For this review, take the finished solid that the model builds, in its own axes (mm). A direction names the side the tool comes from. Coordinates: 2 decimals unless noted, no trailing zeros. Order: outer loops, then holes, each group sorted by start corner. A loop starts at its lowest first (then second) coordinate and runs counter-clockwise, first axis right, second up. Notation, with made-up numbers: (63.5, 3) -> (122.5, 3) arc R13 ccw to (122.5, 28) -> close; hole circle Ø10 at (-35.5, 67). An arc over 180 degrees is marked (long way). Answer as a JSON object with one key per item and string values. Group by question number.
1) Machinability: for faces 4 (the flat face through (6, 7, 3)), 5 (the flat face through (-0.1, 26.5, 0.5)), 6 (the flat face through (0, 12, -6)), which of the approach directions +Z, -Z, +X, -X, +Y, -Y give a long, thin tool a straight path to every point of the face, cutting with its end or side? Answer none if there is none.
2) Add section A-A, the plane z = 2.75. Write out the cut boundary in (x, y).
3) For pin 1 (2 mm diameter, centred on x = 6, y = -6.5, fed in from +Z); pin 2 (2 mm diameter, centred on x = 5.5, y = -6, fed in from -Z); pin 3 (1.6 mm diameter, centred on x = 5.5, y = 5.5, fed in from +Z), all flat-tipped, find the tip position at first contact; note any pin that passes through.
4) Wall thickness on L1, parallel to Y at x = -7, z = -4.25; L2, parallel to X at y = 24, z = 2; L3, parallel to Y at x = -8.25, z = 2: over which ranges is each line inside the solid? List them lowest first.
5) Add section B-B, the plane y = 21. Write out the cut boundary in (x, z), then the cut area to 3 significant figures.
6) Add section D-D, the plane y = -5.5. Write out the cut boundary in (x, z).
7) Draft analysis for pull direction X (two halves, no side actions). For faces 1 (the flat face through (0, 19, -7.5)), 2 (the flat face through (6, -6, -2)), 3 (the flat face through (-12, 0, 0)), state which applies: +X half, -X half, draft (parallel to the pull), parting line (faces both ways), or undercut.
from build123d import *

# Parameters (mm, degrees)
AUFSATZ_LINEAR_AUSTRAGEN1_DEPTH      = 5
AUFSATZ_LINEAR_AUSTRAGEN1_DEPTH_BACK = 5
SKIZZE1_W                            = 24
SKIZZE1_H                            = 24
SKIZZE3_W                            = 15
SKIZZE3_H                            = 15
AUFSATZ_LINEAR_AUSTRAGEN2_DEPTH      = 15
SCHNITT_LINEAR_AUSTRAGEN1_DEPTH      = 10
FASE1_SIZE                           = 1
SCHNITT_LINEAR_START                 = -11
SKIZZE6_W                            = 2
SKIZZE6_H                            = 2
SCHNITT_LINEAR_AUSTRAGEN2_DEPTH      = 12
FASE2_SIZE                           = 1
SKIZZE12_W                           = 15
SKIZZE12_H                           = 15
SCHNITT_LINEAR_AUSTRAGEN4_DEPTH      = 2.5


with BuildPart() as part:
    # Skizze1 → Aufsatz-Linear austragen1 (new, two sides: drawn at the far end of the back side and taken through both)
    with BuildSketch(Plane.XY.offset(-AUFSATZ_LINEAR_AUSTRAGEN1_DEPTH_BACK)):
        Rectangle(SKIZZE1_W, SKIZZE1_H)
    extrude(amount=AUFSATZ_LINEAR_AUSTRAGEN1_DEPTH + AUFSATZ_LINEAR_AUSTRAGEN1_DEPTH_BACK)

    # Skizze3 → Aufsatz-Linear austragen2 (add)
    with BuildSketch(Plane(origin=(0, 12, 0), x_dir=(1, 0, 0), z_dir=(0, 1, 0))):
        Rectangle(SKIZZE3_W, SKIZZE3_H)
    extrude(amount=AUFSATZ_LINEAR_AUSTRAGEN2_DEPTH)

    # Skizze5 → Schnitt-Linear austragen1 (cut)
    with BuildSketch(Plane(origin=(0, 27, 0), x_dir=(1, 0, 0), z_dir=(0, 1, 0))):
        with BuildLine():
            Line((-5.1, 0), (5.1, 0))
            ThreePointArc((5.1, 0), (0, 5.1), (-5.1, 0))
        make_face()
    extrude(amount=-SCHNITT_LINEAR_AUSTRAGEN1_DEPTH, mode=Mode.SUBTRACT)

    # Fase1
    fase1_edges = [part.edges().sort_by_distance(p)[0] for p in [
        (0, 27, -5.1),
        (0, 27, 0),
    ]]
    chamfer(fase1_edges, length=FASE1_SIZE)

    # Skizze6 → Schnitt-Linear austragen2 (cut)
    with BuildSketch(Plane.XY.offset(-3).offset(SCHNITT_LINEAR_START)):
        with Locations((6, 6)):
            Rectangle(SKIZZE6_W, SKIZZE6_H)
        with Locations((6, -6)):
            Rectangle(SKIZZE6_W, SKIZZE6_H)
        with Locations((-6, -6)):
            Rectangle(SKIZZE6_W, SKIZZE6_H)
        with Locations((-6, 6)):
            Rectangle(SKIZZE6_W, SKIZZE6_H)
    schnitt_linear_austragen2 = extrude(amount=SCHNITT_LINEAR_AUSTRAGEN2_DEPTH, mode=Mode.SUBTRACT)

    # Spiegeln1: Schnitt-Linear austragen2 across plane
    add(schnitt_linear_austragen2.mirror(Plane.XY), mode=Mode.SUBTRACT)

    # Fase2
    fase2_edges = [part.edges().sort_by_distance(p)[0] for p in [
        (6, 5, 5),
        (7, 6, 5),
        (6, 7, 5),
        (5, 6, 5),
        (6, -7, 5),
        (7, -6, 5),
        (6, -5, 5),
        (5, -6, 5),
        (-6, -7, 5),
        (-5, -6, 5),
        (-6, -5, 5),
        (-7, -6, 5),
        (-6, 5, 5),
        (-5, 6, 5),
        (-6, 7, 5),
        (-7, 6, 5),
        (6, 7, -5),
        (7, 6, -5),
        (6, 5, -5),
        (5, 6, -5),
        (6, -5, -5),
        (7, -6, -5),
        (6, -7, -5),
        (5, -6, -5),
        (-6, -5, -5),
        (-5, -6, -5),
        (-6, -7, -5),
        (-7, -6, -5),
        (-6, 7, -5),
        (-5, 6, -5),
        (-6, 5, -5),
        (-7, 6, -5),
    ]]
    chamfer(fase2_edges, length=FASE2_SIZE)

    # Skizze12 → Schnitt-Linear austragen4 (cut)
    with BuildSketch(Plane.XY.offset(7.5)):
        with Locations((0, 19.5)):
            Rectangle(SKIZZE12_W, SKIZZE12_H)
    extrude(amount=-SCHNITT_LINEAR_AUSTRAGEN4_DEPTH, mode=Mode.SUBTRACT)


solid = part.part
Output values:
{
 "1": {"face 4": "+Z", "face 5": "+Y", "face 6": "-Z, +X, -X, -Y"},
 "2": {"outline": "(-12, -12) -> (12, -12) -> (12, 12) -> (7.5, 12) -> (7.5, 27) -> (-7.5, 27) -> (-7.5, 12) -> (-12, 12) -> close; hole (-7, -7) -> (-5, -7) -> (-5, -5) -> (-7, -5) -> close; hole (-7, 5) -> (-5, 5) -> (-5, 7) -> (-7, 7) -> close; hole (5, -7) -> (7, -7) -> (7, -5) -> (5, -5) -> close; hole (5, 5) -> (7, 5) -> (7, 7) -> (5, 7) -> close"},
 "3": {"pin 1": "stops at z = 4.5", "pin 2": "stops at z = -4.5", "pin 3": "stops at z = 4.3"},
 "4": {"L1": "y = -12 to -7.25, -4.75 to 4.75, 7.25 to 27", "L2": "x = -7.5 to 7.5", "L3": "y = -12 to 12"},
 "5": {"outline": "(-7.5, -7.5) -> (7.5, -7.5) -> (7.5, 5) -> (-7.5, 5) -> close; hole (-5.1, 0) arc R5.1 ccw to (5.1, 0) -> close", "area": "147 mm²"},
 "6": {"outline": "(-12, -5) -> (-8, -5) -> (-7, -4) -> (-7, -2) -> (-5, -2) -> (-5, -4) -> (-4, -5) -> (4, -5) -> (5, -4) -> (5, -2) -> (7, -2) -> (7, -4) -> (8, -5) -> (12, -5) -> (12, 5) -> (8, 5) -> (7, 4) -> (7, 2) -> (5, 2) -> (5, 4) -> (4, 5) -> (-4, 5) -> (-5, 4) -> (-5, 2) -> (-7, 2) -> (-7, 4) -> (-8, 5) -> (-12, 5) -> close"},
 "7": {"face 1": "draft", "face 2": "undercut", "face 3": "-X half"}
}
